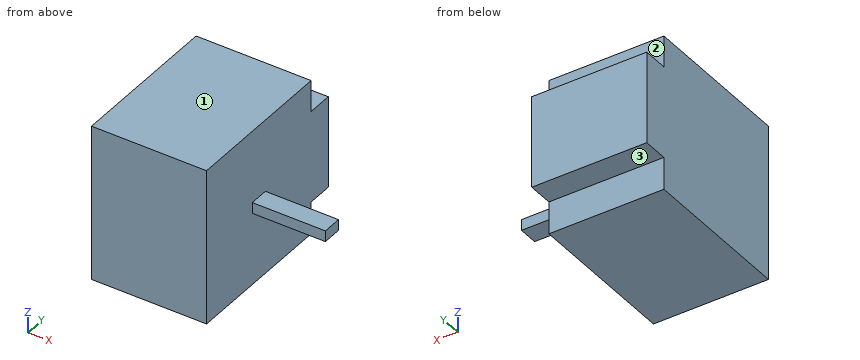
```python
from build123d import *

# Parameters (mm, degrees)
SKETCH1_W           = 16
SKETCH1_H           = 16
SKETCH1_W_2         = 9.45
SKETCH1_H_2         = 2.62
BOSS_EXTRUDE3_DEPTH = 11.8
SKETCH2_W           = 1.12
SKETCH2_H           = 2
BOSS_EXTRUDE4_DEPTH = 7.5


with BuildPart() as part:
    # Sketch1 → Boss-Extrude3 (new body)
    with BuildSketch(Plane(origin=(0, 0, 0), x_dir=(0, 0, -1), z_dir=(1, 0, 0))):
        with Locations((8, 8)):
            Rectangle(SKETCH1_W, SKETCH1_H)
        with Locations((7.95, 17.31)):
            Rectangle(SKETCH1_W_2, SKETCH1_H_2)
    extrude(amount=BOSS_EXTRUDE3_DEPTH)

    # Sketch2 → Boss-Extrude4 (add)
    with BuildSketch(Plane(origin=(11.8, 0, 0), x_dir=(0, 0, -1), z_dir=(1, 0, 0))):
        with Locations((8, 8)):
            Rectangle(SKETCH2_W, SKETCH2_H)
    extrude(amount=BOSS_EXTRUDE4_DEPTH)


solid = part.part
```
Geometry: final body of the model. Coordinates: model frame, mm. Face numbers are marked on the shaded views. A direction names the side the tool comes from. Give positions to 0.01 mm unless a question says otherwise; leave off trailing zeros. Loops run counter-clockwise (first coordinate to the right, second up) from the corner with the lowest first, then second, coordinate; pieces in that order, holes last. Notation, with made-up numbers: (74.25, 11) -> (116.25, 11) arc R29 cw to (116.25, 35) -> close; hole circle Ø5 at (-16, 48). An arc over 180 degrees is marked (long way). Use CSV: the item, a comma, the result in double quotes.
(1) Cut plane B-B (x = 2.25). Output: boundary loops of the cut face in (y, z) (3 decimals), plus the area to 3 significant figures.
From the geometry:
outline,"(0, -16) -> (16, -16) -> (16, -12.675) -> (18.62, -12.675) -> (18.62, -3.225) -> (16, -3.225) -> (16, 0) -> (0, 0) -> close"
area,"281 mm^2"
(2) First-contact query: P1, Ø0.8, axis at x = 3, y = 17, coming from the -Z side (3 decimals); P2, Ø0.6, axis at x = 14.5, y = 8, coming from the -Z side; P3, Ø1.7, axis at x = 4, z = -14.5, coming from the +Y side. Flat tips, straight axial feed; report the tip coordinate or a pass-through.
From the geometry:
P1,"z = -12.675"
P2,"z = -8.56"
P3,"y = 16"
(3) Access query for the marked faces 1, 2 and 3. Directions: +Z, -Z, +X, -X, +Y, -Y. A direction counts if a zero-diameter tool reaches every point of the face in a straight line with its end or side. Return the directions, or none.
From the geometry:
face 1,"+Z, +X, -X, +Y, -Y"
face 2,"+Z, +X, -X, +Y"
face 3,"-Z, +X, -X, +Y"
(4) Cut plane D-D (y = 17.5). Output: boundary loops of the cut face in (x, z) (3 decimals), plus the area to 3 significant figures.
From the geometry:
outline,"(0, -12.675) -> (11.8, -12.675) -> (11.8, -3.225) -> (0, -3.225) -> close"
area,"112 mm^2"
(5) Cut plane A-A (y = 8.5). Output: boundary loops of the cut face in (x, z), plus the area to 3 significant figures.
From the geometry:
outline,"(0, -16) -> (11.8, -16) -> (11.8, -8.56) -> (19.3, -8.56) -> (19.3, -7.44) -> (11.8, -7.44) -> (11.8, 0) -> (0, 0) -> close"
area,"197 mm^2"
(6) Cut plane C-C (z = -4.5). Output: boundary loops of the cut face in (x, y), plus the area to 3 significant figures.
From the geometry:
outline,"(0, 0) -> (11.8, 0) -> (11.8, 18.62) -> (0, 18.62) -> close"
area,"220 mm^2"
(7) Ray query, line 1 along X through (y, z) = (1, -13.25); line 2 along Y through (x, z) = (2.75, -3). Return the intervals inside material, ascending. Write a range as [from, to].
From the geometry:
line 1,"[0, 11.8]"
line 2,"[0, 16]"
